Work out the finished part from the listing and answer in its coordinate system (mm). A direction names the side the tool comes from. Coordinates: 2 decimals unless noted, no trailing zeros. Write each loop counter-clockwise with the first axis right and the second up, starting at its lowest first coordinate (ties: lowest second). Pieces come first, ordered by that corner, then holes. Notation, with made-up numbers: (-24.75, -25) - (-11.75, -25) arc R13 ccw to (-11.75, 0) - close; hole circle Ø8 at (-16, 10.25). An arc over 180 degrees is marked (long way). One line per item, written item: value.
```python
from build123d import *

# Parameters (mm, degrees)
SKETCH1_R           = 4.826
SKETCH1_R_2         = 4.064
SKETCH3_R           = 4.826
BOSS_EXTRUDE1_DEPTH = 2.54
BOSS_EXTRUDE1_DRAFT = -37
SKETCH5_R           = 4.826
BOSS_EXTRUDE2_DEPTH = 2.54
BOSS_EXTRUDE2_DRAFT = -37


with BuildPart() as part:
    # Sweep1: sweep along a path in Sketch2
    with BuildLine(Plane.XY) as sweep1_path:
        Line((0, 0), (0, 206.956941604))
        ThreePointArc((0, 206.956941604), (0.649113009, 211.887444413), (2.552216058, 216.481941604))
        Line((2.552216058, 216.481941604), (47.002216058, 293.4716))
    # Sketch1 → Sweep1 (sweep)
    with BuildSketch(Plane(origin=(0, 0, 0), x_dir=(1, 0, 0), z_dir=(0, 1, 0))):
        Circle(SKETCH1_R)
        Circle(SKETCH1_R_2, mode=Mode.SUBTRACT)
    sweep(path=sweep1_path.line)


with BuildPart() as boss_extrude1_tool:
    # Sketch3 → Boss-Extrude1 (with draft: the straight prism first)
    with BuildSketch(Plane.XZ):
        with Locations(Location((0, 0, 0), (0, 0, 180))):
            Circle(SKETCH3_R)
    extrude(amount=BOSS_EXTRUDE1_DEPTH)
    # Boss-Extrude1: the draft: its side faces are tilted about the plane it starts from
    boss_extrude1_sides = [boss_extrude1_tool.faces().sort_by_distance(p)[0] for p in [
        (4.826, -1.27, 0),
    ]]
    draft(boss_extrude1_sides, Plane.XZ, BOSS_EXTRUDE1_DRAFT)


with BuildPart() as part_1:
    add(part.part)

    # Boss-Extrude1: add boss_extrude1_tool
    add(boss_extrude1_tool.part)

    # Cut-Extrude1 cone 1 section (through the dimple's axis) → Cut-Extrude1 (revolve, cut)
    with BuildSketch(Plane(origin=(0, -2.54, 0), x_dir=(0, 0, -1), z_dir=(1, 0, 0))):
        Polygon((0, 0), (5.978027287, 0), (0, 7.933110155), align=None)
    revolve(axis=Axis((0, -2.54, 0), (0, 1, 0)), mode=Mode.SUBTRACT)


with BuildPart() as boss_extrude2_tool:
    # Sketch5 → Boss-Extrude2 (with draft: the straight prism first)
    with BuildSketch(Plane(origin=(138.827484459, 240.45625657, 0), x_dir=(0, 0, -1), z_dir=(0.5000000000000008, 0.8660254037844382, 0))):
        with Locations(Location((0, 106.03068686, 0), (0, 0, 90))):
            Circle(SKETCH5_R)
    extrude(amount=BOSS_EXTRUDE2_DEPTH)
    # Boss-Extrude2: the draft: its side faces are tilted about the plane it starts from
    boss_extrude2_sides = [boss_extrude2_tool.faces().sort_by_distance(p)[0] for p in [
        (51.816654657, 292.158452263, 0),
    ]]
    draft(boss_extrude2_sides, Plane(origin=(138.827484459, 240.45625657, 0), x_dir=(0, 0, -1), z_dir=(0.5000000000000008, 0.8660254037844382, 0)), BOSS_EXTRUDE2_DRAFT)


with BuildPart() as part_2:
    add(part_1.part)

    # Boss-Extrude2: add boss_extrude2_tool
    add(boss_extrude2_tool.part)

    # Cut-Extrude2 cone 1 section (through the dimple's axis) → Cut-Extrude2 (revolve, cut)
    with BuildSketch(Plane(origin=(48.272216058, 295.671304526, 0), x_dir=(0, 0, 1), z_dir=(0.866025404, -0.5, 0))):
        Polygon((0, 0), (5.978027287, 0), (0, 7.933110155), align=None)
    revolve(axis=Axis((48.272216058, 295.671304526, 0), (-0.5, -0.866025404, 0)), mode=Mode.SUBTRACT)


solid = part_2.part
```
Item 1: Given pin 1 (6 mm diameter, centred on y = 87, z = -4, fed in from -X); pin 2 (2 mm diameter, centred on x = 2, z = 0, fed in from -Y); pin 3 (6 mm diameter, centred on y = 146, z = 1.5, fed in from -X), each flat-ended and moving along its own axis, determine where each tip first touches the part or whether it passes through.
Evaluation:
pin 1: stops at x = -4.72
pin 2: stops at y = 221.92
pin 3: stops at x = -4.83
Item 2: Consider probe 1 along Z at (x, y) = (0, 119); probe 2 along Z at (x, y) = (-3.5, 47). Determine where each line is inside the solid, lowest interval first.
Evaluation:
probe 1: z = -4.83 to -4.06, 4.06 to 4.83
probe 2: z = -3.32 to -2.07, 2.07 to 3.32
Item 3: Which of the six approach directions +Z, -Z, +X, -X, +Y, -Y give full straight-line access (tool end or side, diameter ignored) to faces 5 (the face through (1.07, -0.12, 4.8)), 6 (the face through (-0.881, 104.927, 3.967)), 7 (the face through (4, -2.54, 5))?
Evaluation:
face 5: none
face 6: -Y
face 7: +Z, -Z, +X, -X, -Y
Item 4: Section B-B, the plane y = 81 is taken. Determine the outline of the cut face in (x, z), then the cut area to 3 significant figures.
Evaluation:
outline: circle Ø9.65 at (0, 0); hole circle Ø8.13 at (0, 0)
area: 21.3 mm2
Item 5: Determine the mould class of faces 1 (the face through (45.983, 294.203, 3.965)), 2 (the face through (28.34, 253.64, 1.56)), 3 (the face through (-1.249, -0.123, -3.965)), 4 (the face through (-3.83, 104.927, 2.937)) for opening direction Y: +Y half, -Y half, draft (parallel to the pull), parting line (faces both ways), or undercut.
Evaluation:
face 1: +Y half
face 2: undercut
face 3: -Y half
face 4: undercut
Item 6: Section A-A, the plane z = 0 is taken. Determine the outline of the cut face in (x, y).
Evaluation:
outline: (-6.74, -2.54) - (-5.98, -2.54) - (-4.06, 0) - (-4.06, 206.96) arc R23.11 cw to (-0.97, 218.51) - (43.48, 295.5) - (43.1, 298.66) - (42.44, 299.04) - (42.82, 295.88) - (-1.63, 218.89) arc R23.88 ccw to (-4.83, 206.96) - (-4.83, 0) - close; (4.06, 0) - (5.98, -2.54) - (6.74, -2.54) - (4.83, 0) - (4.83, 206.96) arc R14.22 cw to (6.73, 214.07) - (51.18, 291.06) - (54.11, 292.3) - (53.45, 292.68) - (50.52, 291.44) - (6.07, 214.45) arc R14.99 ccw to (4.06, 206.96) - close
